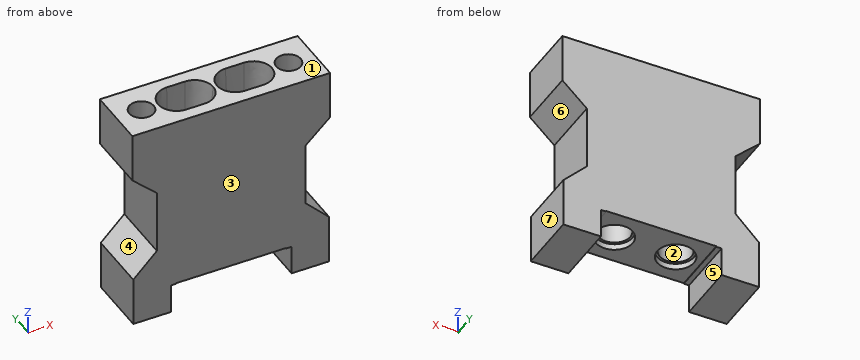
from build123d import *

# Parameters (mm, degrees)
SKETCH079_R     = 2.7
PAD033_DEPTH    = 10
SKETCH076_R     = 2.6
POCKET031_DEPTH = 8
SKETCH077_R     = 3
POCKET032_DEPTH = 1
SKETCH080_R     = 2
POCKET033_DEPTH = 8


with BuildPart() as loft005:
    # Sketch079 → Loft005 section 0
    with BuildSketch(Plane.XY.offset(16)):
        with Locations((-5, 0)):
            Circle(SKETCH079_R)
    # Sketch078 → Loft005 section 1
    with BuildSketch(Plane.XY.offset(38)):
        with BuildLine():
            ThreePointArc((-6.3, 3), (-9.3, 0), (-6.3, -3))
            Line((-6.3, -3), (-3.3, -3))
            ThreePointArc((-3.3, -3), (-0.3, 0), (-3.3, 3))
            Line((-3.3, 3), (-6.3, 3))
        make_face()
    loft()


with BuildPart() as part_mirroring005:
    # Part__Mirroring005: instance of Loft005
    add(loft005.part.mirror(Plane(origin=(0, 0, 0), x_dir=(0, -1, 0), z_dir=(1, 0, 0))))


with BuildPart() as fusion005:
    # Fusion005 base: copy of Loft005
    add(loft005.part)

    # Fusion005: union Part__Mirroring005
    add(part_mirroring005.part)


with BuildPart() as fusion005_1:
    # Fusion005 placement: moved
    add(fusion005.part.moved(Location((0, -5, 0))))


with BuildPart() as cut004:
    # Sketch075 → Pad033 (new body)
    with BuildSketch(Plane.XZ):
        Polygon((-16, 4), (-9.85, 4), (-9.85, 7.2), (-9.85, 8.8), (-9, 8.8), (-9, 8.9), (9, 8.9), (9, 8.8), (9.85, 8.8), (9.85, 7.2), (9.85, 4), (16, 4), (16, 12), (12.15, 15.85), (12.15, 26.306086), (16.15, 30), (16.15, 38), (-16.15, 38), (-16.15, 30), (-12.15, 26.306086), (-12.15, 15.85), (-16, 12), align=None)
    extrude(amount=PAD033_DEPTH)

    # Sketch076 (on Face7 of Pad033) → Pocket031 (cut)
    with BuildSketch(Plane(origin=(0, 0, 8.9), x_dir=(1, 0, 0), z_dir=(0, 0, -1))):
        with Locations((-5, 5)):
            Circle(SKETCH076_R)
        with Locations((5, 5)):
            Circle(SKETCH076_R)
    extrude(amount=-POCKET031_DEPTH, mode=Mode.SUBTRACT)

    # Sketch077 (on Face11 of Pocket031) → Pocket032 (cut)
    with BuildSketch(Plane(origin=(0, 0, 8.9), x_dir=(1, 0, 0), z_dir=(0, 0, -1))):
        with Locations((-5, 5)):
            Circle(SKETCH077_R)
        with Locations((5, 5)):
            Circle(SKETCH077_R)
    extrude(amount=-POCKET032_DEPTH, mode=Mode.SUBTRACT)

    # Sketch080 (on Face22 of Pocket032) → Pocket033 (cut)
    with BuildSketch(Plane(origin=(0, 0, 38), x_dir=(-1, 0, 0), z_dir=(0, 0, 1))):
        with Locations((-12, 5)):
            Circle(SKETCH080_R)
        with Locations((12, 5)):
            Circle(SKETCH080_R)
    extrude(amount=-POCKET033_DEPTH, mode=Mode.SUBTRACT)

    # Cut004: cut Fusion005
    add(fusion005_1.part, mode=Mode.SUBTRACT)


with BuildPart() as cut004_1:
    # Cut004 placement: moved
    add(cut004.part.moved(Location((0, -474.33, 0))))


solid = cut004_1.part
Source: CAD feature listing. Evaluate the final solid. Frame: model axes, mm. Face numbers are marked on the shaded views. A direction names the side the tool comes from. Round coordinates to 2 decimals unless told otherwise and drop trailing zeros. Loops run counter-clockwise (first coordinate to the right, second up) from the corner with the lowest first, then second, coordinate; pieces in that order, holes last. Notation, with made-up numbers: (74, 38) - (115, 38) arc R18 cw to (115, 42) - close; hole circle Ø8 at (-5.5, 44). An arc over 180 degrees is marked (long way). Write item = value, one per line. Start each with the question number.
Item 1: Section query B-B on y = -475. Output: boundary loops of the cut face in (x, z), plus the area to 3 significant figures.
Item 2: First-contact query: pin 1 Ø3 at (x, y) = (4.5, -478) entering from -Z; pin 2 Ø4 at (y, z) = (-481.5, 5.5) entering from +X; pin 3 Ø1.6 at (x, y) = (5, -480.5) entering from +Z; pin 4 Ø5 at (x, y) = (-3.5, -480) entering from -Z. Flat tips, straight axial feed; report the tip coordinate or a pass-through.
Item 3: Reachability of the marked faces 4, 5, 6 and 7 from +Z, -Z, +X, -X, +Y, -Y: full face, straight path, thin tool, end or side. Return the list, or none.
Item 4: Section query A-A on x = -13. Output: boundary loops of the cut face in (y, z), plus the area to 3 significant figures.
Item 5: Mould query, pull axis Y, two halves, no side actions, for the marked faces 1, 2 and 3. Classes: released by +Y, released by -Y, zero draft, split by the parting line, or undercut.
Item 6: Section query D-D on x = 10.5. Output: boundary loops of the cut face in (y, z), plus the area to 3 significant figures.
Item 7: Material intervals for line 1 (Y direction, x = 5, z = 14); line 2 (X direction, y = -479.33, z = 9.6); line 3 (Y direction, x = 5, z = 9.4), sorted ascending.
Item 8: Section query C-C on z = 22. Count the separate pieces of the cut face and the enclosed holes in it, plus the area to 3 significant figures.
Results list:
q1.outline = (-16.15, 30) - (-12.15, 26.31) - (-12.15, 15.85) - (-16, 12) - (-16, 4) - (-9.85, 4) - (-9.85, 8.8) - (-9, 8.8) - (-9, 8.9) - (9, 8.9) - (9, 8.8) - (9.85, 8.8) - (9.85, 4) - (16, 4) - (16, 12) - (12.15, 15.85) - (12.15, 26.31) - (16.15, 30) - (16.15, 38) - (-16.15, 38) - close
q1.area = 885 mm²
q2.pin_1 = 9.9
q2.pin_2 = 16
q2.pin_3 = through
q2.pin_4 = 8.9
q3.face_4 = -X, +Y, -Y
q3.face_5 = -Z, +Y, -Y
q3.face_6 = +X, +Y, -Y
q3.face_7 = -Z, +X, +Y, -Y
q4.outline = (-484.33, 4) - (-474.33, 4) - (-474.33, 15) - (-484.33, 15) - close; (-484.33, 27.09) - (-474.33, 27.09) - (-474.33, 38) - (-477.6, 38) - (-477.6, 30) - (-481.06, 30) - (-481.06, 38) - (-484.33, 38) - close
q4.area = 191 mm²
q5.face_1 = zero draft
q5.face_2 = undercut
q5.face_3 = released by -Y
q6.outline = (-484.33, 4) - (-474.33, 4) - (-474.33, 38) - (-478.01, 38) - (-478.01, 30) - (-480.65, 30) - (-480.65, 38) - (-484.33, 38) - close
q6.area = 319 mm²
q7.line_1 = -484.33 to -481.93, -476.73 to -474.33
q7.line_2 = -16 to -8, -2 to 2, 8 to 16
q7.line_3 = -484.33 to -482.33, -476.33 to -474.33
q8.separate_pieces = 1
q8.enclosed_holes = 2
q8.area = 186 mm²
